Build history of the part. All positions in model axes, mm. Face numbers are marked on the shaded views. A direction names the side the tool comes from. Coordinates: 2 decimals unless noted, no trailing zeros. Order: outer loops, then holes, each group sorted by start corner. A loop starts at its lowest first (then second) coordinate and runs counter-clockwise, first axis right, second up. Notation, with made-up numbers: (23, 47) - (35, 47) arc R21 ccw to (35, 77) - close; hole circle Ø1 at (78.25, -13). An arc over 180 degrees is marked (long way). Return JSON: item names as keys, results as strings.
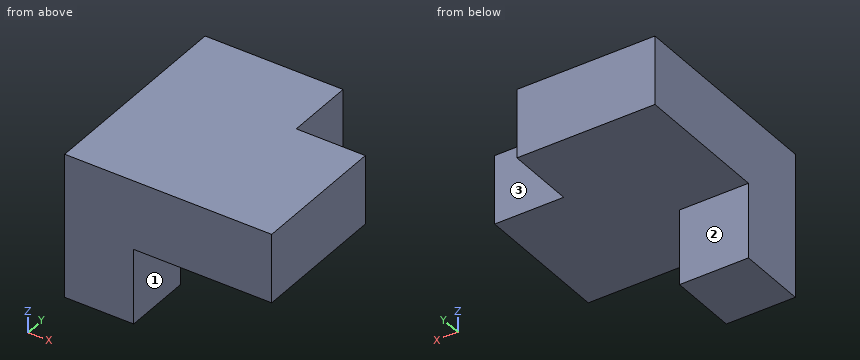
from build123d import *

# Parameters (mm, degrees)
F0_W     = 76.2
F0_H     = 76.2
F1_DEPTH = 25.4
F2_W     = 25.4
F2_H     = 25.4
F3_DEPTH = 25.4
F4_W     = 25.4
F4_H     = 25.4
F5_DEPTH = 27.686


with BuildPart() as f1:
    # F0 (on Top) → F1 (new body)
    with BuildSketch(Plane.XY):
        with Locations((38.1, 38.1)):
            Rectangle(F0_W, F0_H)
    extrude(amount=F1_DEPTH)

    # F2 (on face) → F3 (cut)
    with BuildSketch(Plane.XY.offset(25.4)):
        with Locations((63.5, 63.5)):
            Rectangle(F2_W, F2_H)
    extrude(amount=-F3_DEPTH, mode=Mode.SUBTRACT)

    # F4 (on Top) → F5 (join)
    with BuildSketch(Plane.XY):
        with Locations((12.7, 12.7)):
            Rectangle(F4_W, F4_H)
    extrude(amount=-F5_DEPTH)


solid = f1.part
1. Cut at B-B on y = 5. Give the cut face in (x, z), plus the area to 3 significant figures.
Check values:
{"outline": "(0, -27.69) - (25.4, -27.69) - (25.4, 0) - (76.2, 0) - (76.2, 25.4) - (0, 25.4) - close", "area": "2,640 mm²"}
2. Cut at A-A on z = 11. Give the cut face in (x, y), plus the area to 3 significant figures.
Check values:
{"outline": "(0, 0) - (76.2, 0) - (76.2, 50.8) - (50.8, 50.8) - (50.8, 76.2) - (0, 76.2) - close", "area": "5,160 mm²"}
3. Cut at C-C on x = 63. Give the cut face in (y, z), plus the area to 3 significant figures.
Check values:
{"outline": "(0, 0) - (50.8, 0) - (50.8, 25.4) - (0, 25.4) - close", "area": "1,290 mm²"}
4. Cut at D-D on y = 40.5. Give the cut face in (x, z), plus the area to 3 significant figures.
Check values:
{"outline": "(0, 0) - (76.2, 0) - (76.2, 25.4) - (0, 25.4) - close", "area": "1,940 mm²"}
5. Probe L1, parallel to Y at x = 23, z = -1; L2, parallel to X at y = 57.5, z = 8.5. List the from-to ranges inside material, lowest first.
Check values:
{"L1": "0 to 25.4", "L2": "0 to 50.8"}
6. Drop flat-ended pins along their axis: pin 1 (7.5 mm diameter, centred on x = 69, z = 8.5, fed in from +Y); pin 2 (4 mm diameter, centred on y = 60, z = 5.5, fed in from +X); pin 3 (20.5 mm diameter, centred on x = 14.5, z = -20, fed in from +Y). Give the stop position or say it passes through.
Check values:
{"pin 1": "y = 50.8", "pin 2": "x = 50.8", "pin 3": "y = 25.4"}
7. Tool access for the marked faces 1, 2 and 3: list every direction of +Z, -Z, +X, -X, +Y, -Y with a clear straight run to the whole face (end or side of a thin tool).
Check values:
{"face 1": "-Z, +X, +Y, -Y", "face 2": "-Z, +X, -X, +Y", "face 3": "+Z, -Z, +X, +Y"}
